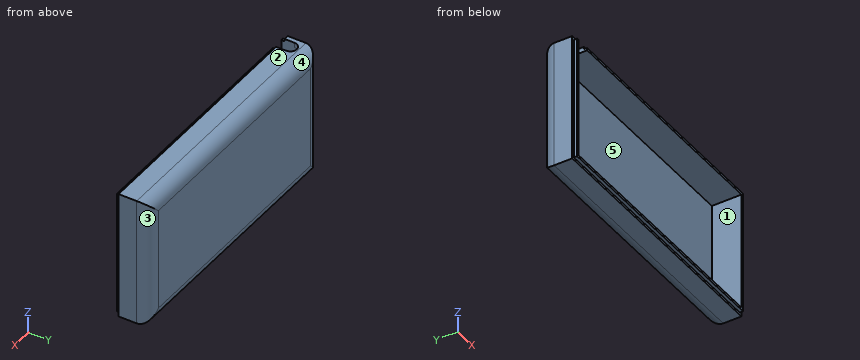
from build123d import *

# Parameters (mm, degrees)
SKETCH1_W           = 80
SKETCH1_H           = 39
SKETCH1_W_2         = 77
SKETCH1_H_2         = 36
BOSS_EXTRUDE1_DEPTH = 9
SKETCH2_W           = 80
SKETCH2_H           = 39
BOSS_EXTRUDE2_DEPTH = 1.5
SKETCH4_W           = 80
SKETCH4_H           = 39
SKETCH4_W_2         = 78.5
SKETCH4_H_2         = 37.5
CUT_EXTRUDE1_DEPTH  = 1
FILLET1_R           = 4
CUT_EXTRUDE2_REACH  = 58.844


with BuildPart() as part:
    # Sketch1 → Boss-Extrude1 (new body)
    with BuildSketch(Plane(origin=(0, 0, 0), x_dir=(1, 0, 0), z_dir=(0, 1, 0))):
        Rectangle(SKETCH1_W, SKETCH1_H)
        Rectangle(SKETCH1_W_2, SKETCH1_H_2, mode=Mode.SUBTRACT)
    extrude(amount=BOSS_EXTRUDE1_DEPTH)

    # Sketch2 → Boss-Extrude2 (add)
    with BuildSketch(Plane(origin=(0, 9, 0), x_dir=(1, 0, 0), z_dir=(0, 1, 0))):
        Rectangle(SKETCH2_W, SKETCH2_H)
    extrude(amount=BOSS_EXTRUDE2_DEPTH)

    # Sketch4 → Cut-Extrude1 (cut)
    with BuildSketch(Plane.XZ):
        Rectangle(SKETCH4_W, SKETCH4_H)
        Rectangle(SKETCH4_W_2, SKETCH4_H_2, mode=Mode.SUBTRACT)
    extrude(amount=-CUT_EXTRUDE1_DEPTH, mode=Mode.SUBTRACT)

    # Fillet1
    fillet1_edges = [part.edges().sort_by_distance(p)[0] for p in [
        (-40, 10.5, 0),
        (0, 10.5, 19.5),
        (40, 10.5, 0),
        (0, 10.5, -19.5),
    ]]
    fillet(fillet1_edges, radius=FILLET1_R)

    # Sketch5 → Cut-Extrude2 (cut, up to next)
    with BuildSketch(Plane.XY.offset(19.5), mode=Mode.PRIVATE) as cut_extrude2_sk1:
        with BuildLine():
            Line((-38.5, -2), (-38.5, 4))
            ThreePointArc((-38.5, 4), (-36.5, 6), (-34.5, 4))
            Line((-34.5, 4), (-34.5, -2))
            ThreePointArc((-34.5, -2), (-36.5, -4), (-38.5, -2))
        make_face()
    cut_extrude2_tool1 = extrude(cut_extrude2_sk1.sketch, amount=-CUT_EXTRUDE2_REACH, mode=Mode.PRIVATE) & part.part
    add(cut_extrude2_tool1.solids().sort_by_distance((-36.5, 1, 19.5))[0], mode=Mode.SUBTRACT)


solid = part.part
Model file for the job. Use its own axes, mm. Face numbers are marked on the shaded views. A direction names the side the tool comes from. Round coordinates to 2 decimals unless told otherwise and drop trailing zeros. Loops run counter-clockwise (first coordinate to the right, second up) from the corner with the lowest first, then second, coordinate; pieces in that order, holes last. Notation, with made-up numbers: (-15.75, 47) -> (10.25, 47) arc R3 ccw to (10.25, 52) -> close; hole circle Ø6 at (-39, 61.25). An arc over 180 degrees is marked (long way). Answer as CSV lines item,"result". Start each with the question number.
1) Mould opens along Z. For the marked faces 3, 4 and 5 say: +Z half, -Z half, draft (parallel to the pull), parting line (faces both ways), or undercut.
2) Slice it at B-B (x = -17). List the corners of the cut face in (y, z), plus the area to 3 significant figures.
3) Slice it at C-C (y = 8.25). List the corners of the cut face in (x, z), plus the area to 3 significant figures.
4) Slice it at A-A (z = 7). List the corners of the cut face in (x, y).
5) Pin check, flat tips, straight feed: P1, Ø18, axis at x = -3.5, z = -8.5, coming from the -Y side; P2, Ø0.8, axis at x = -39, y = 0.5, coming from the +Z side; P3, Ø0.8, axis at x = 1.5, y = 0.5, coming from the -Z side. Stop position of each tip, or through.
6) Probe line 1 along Z through (x, y) = (18.5, 3.5); line 2 along X through (y, z) = (3, -15.5); line 3 along Z through (x, y) = (5.5, 0.75). List the from-to ranges inside material, lowest first.
7) Tool access for the marked faces 1 and 2: list every direction of +Z, -Z, +X, -X, +Y, -Y with a clear straight run to the whole face (end or side of a thin tool).
Filled in:
1,face 3,"draft"
1,face 4,"+Z half"
1,face 5,"undercut"
2,outline,"(0, -18.75) -> (1, -18.75) -> (1, -19.5) -> (6.5, -19.5) arc R4 ccw to (10.5, -15.5) -> (10.5, 15.5) arc R4 ccw to (6.5, 19.5) -> (1, 19.5) -> (1, 18.75) -> (0, 18.75) -> (0, 18) -> (9, 18) -> (9, -18) -> (0, -18) -> close"
2,area,"77.1 mm2"
3,outline,"(-39.6, -19.1) -> (39.6, -19.1) -> (39.6, 19.1) -> (-39.6, 19.1) -> close; hole (-38.5, -18) -> (38.5, -18) -> (38.5, 18) -> (-38.5, 18) -> close"
3,area,"253 mm2"
4,outline,"(-40, 1) -> (-39.25, 1) -> (-39.25, 0) -> (-38.5, 0) -> (-38.5, 9) -> (38.5, 9) -> (38.5, 0) -> (39.25, 0) -> (39.25, 1) -> (40, 1) -> (40, 6.5) arc R4 ccw to (36, 10.5) -> (-36, 10.5) arc R4 ccw to (-40, 6.5) -> close"
5,P1,"stops at y = 9"
5,P2,"stops at z = 18.75"
5,P3,"stops at z = -18.75"
6,line 1,"z = -19.5 to -18, 18 to 19.5"
6,line 2,"x = -40 to -38.5, 38.5 to 40"
6,line 3,"z = -18.75 to -18, 18 to 18.75"
7,face 1,"-Y"
7,face 2,"+Z, +X, -X, +Y, -Y"
